Verification items for the finished model (mm, model axes). A direction names the side the tool comes from. Round coordinates to 2 decimals unless told otherwise and drop trailing zeros. Write each loop counter-clockwise with the first axis right and the second up, starting at its lowest first coordinate (ties: lowest second). Pieces come first, ordered by that corner, then holes. Notation, with made-up numbers: (47, 41) - (52, 41) arc R24 ccw to (52, 77) - close; hole circle Ø9 at (20.25, 39.5). An arc over 180 degrees is marked (long way). Write each question's results on one line, items separated by ' | '.
```python
from build123d import *

# Parameters (mm, degrees)
SKETCH1_W               = 25.4
SKETCH1_H               = 10.16
REVOLVE1_ANGLE          = 180
SKETCH4_W               = 6.29000012
SKETCH4_H               = 3.69
SKETCH6_W               = 3.294985449
SKETCH6_H               = 5.974962046
BOSS_EXTRUDE1_DEPTH     = 5.08
SKETCH7_R               = 3.22
BOSS_EXTRUDE7_DEPTH     = 12.7
SKETCH9_W               = 3.294985449
SKETCH9_H               = 5.974962046
BOSS_EXTRUDE8_DEPTH     = 3.302
CUT_EXTRUDE1_DEPTH      = 3.302
CUT_EXTRUDE1_DEPTH_BACK = 3.302
SKETCH11_R              = 2.375
CUT_EXTRUDE2_DEPTH      = 2.54
CUT_EXTRUDE2_DEPTH_BACK = 12.446
BOSS_EXTRUDE14_DEPTH    = 3.81
SKETCH15_R              = 2.375
CUT_EXTRUDE3_DEPTH      = 22.352


with BuildPart() as part:
    # Sketch1 → Revolve1 (revolve)
    with BuildSketch(Plane(origin=(0, 0, 0), x_dir=(1, 0, 0), z_dir=(0, 1, 0))):
        with Locations((12.7, 5.451011236)):
            Rectangle(SKETCH1_W, SKETCH1_H)
    revolve(axis=Axis((0, 0, -0.371011236), (1, 0, 0)), revolution_arc=REVOLVE1_ANGLE)

    # Sweep1: sweep along a path in Sketch5
    with BuildLine(Plane.XY) as sweep1_path:
        ThreePointArc((12.7, 0), (20.315428689, -15.331843414), (12.392600359, -30.5071183))
    # Sketch4 → Sweep1 (sweep)
    with BuildSketch(Plane(origin=(0, 0, 0), x_dir=(1, 0, 0), z_dir=(0, 1, 0))):
        with Locations((12.7, 0.371011236)):
            Rectangle(SKETCH4_W, SKETCH4_H)
    sweep(path=sweep1_path.line)

    # Sketch6 → Boss-Extrude1 (add)
    with BuildSketch(Plane(origin=(20.164340987, -6.538110874, 0), x_dir=(0, 0, 1), z_dir=(-0.95124601, 0.308433183, 0))):
        with Locations((-0.361104817, -25.204906835)):
            Rectangle(SKETCH6_W, SKETCH6_H)
    extrude(amount=BOSS_EXTRUDE1_DEPTH)

    # Sketch7 → Boss-Extrude7 (add)
    with BuildSketch(Plane(origin=(15.332011256, -4.971270302, 0), x_dir=(0, 0, 1), z_dir=(-0.95124601, 0.308433183, 0))):
        with Locations((-0.361104816, -31.160979548)):
            Circle(SKETCH7_R)
    extrude(amount=-BOSS_EXTRUDE7_DEPTH)

    # Sketch9 → Boss-Extrude8 (add)
    with BuildSketch(Plane(origin=(15.332011256, -4.971270302, 0), x_dir=(0, 0, 1), z_dir=(-0.95124601, 0.308433183, 0))):
        with Locations((-0.361104817, -25.204906835)):
            Rectangle(SKETCH9_W, SKETCH9_H)
    extrude(amount=BOSS_EXTRUDE8_DEPTH)

    # Sketch10 → Cut-Extrude1 (cut, two sides)
    with BuildSketch(Plane.XY) as cut_extrude1_sk:
        with BuildLine():
            Line((3.495528998, -30.770720391), (5.338405562, -25.087061585))
            Line((5.338405562, -25.087061585), (13.311749617, -27.672348528))
            add(Edge.make_bspline(
                [(13.311749617, -27.672348528), (8.683653097, -30.129373505), (3.495528998, -30.770720391)],
                knots=[0, 0, 0, 1, 1, 1], degree=2))
        make_face()
    extrude(amount=CUT_EXTRUDE1_DEPTH, mode=Mode.SUBTRACT)
    extrude(cut_extrude1_sk.sketch, amount=-CUT_EXTRUDE1_DEPTH_BACK, mode=Mode.SUBTRACT)

    # Sketch11 → Cut-Extrude2 (cut, two sides)
    with BuildSketch(Plane(origin=(27.412835582, -8.888371731, 0), x_dir=(0, 0, -1), z_dir=(0.95124601, -0.308433183, 0))) as cut_extrude2_sk:
        with Locations((0.39169909, -31.12675273)):
            Circle(SKETCH11_R)
    extrude(amount=CUT_EXTRUDE2_DEPTH, mode=Mode.SUBTRACT)
    extrude(cut_extrude2_sk.sketch, amount=-CUT_EXTRUDE2_DEPTH_BACK, mode=Mode.SUBTRACT)

    # Sketch13 → Boss-Extrude14 (add)
    with BuildSketch(Plane(origin=(27.412835582, -8.888371731, 0), x_dir=(0, 0, -1), z_dir=(0.95124601, -0.308433183, 0))):
        with BuildLine():
            Line((6.519856112, -42.694953789), (3.125271975, -32.910924296))
            Line((3.125271975, -32.910924296), (0.972674671, -34.333593678))
            Line((0.972674671, -34.333593678), (4.157973921, -43.514412461))
            ThreePointArc((4.157973921, -43.514412461), (4.274214649, -43.645179802), (4.448875729, -43.655451668))
            Line((4.448875729, -43.655451668), (6.378816905, -42.985855597))
            ThreePointArc((6.378816905, -42.985855597), (6.509584246, -42.869614869), (6.519856112, -42.694953789))
        make_face()
        with BuildLine():
            Line((4.098849122, -37.242411221), (5.662835166, -41.750205096))
            ThreePointArc((5.662835166, -41.750205096), (5.6525633, -41.924866176), (5.521795959, -42.041106905))
            Line((5.521795959, -42.041106905), (4.53660766, -42.382919506))
            ThreePointArc((4.53660766, -42.382919506), (4.361946579, -42.37264764), (4.245705851, -42.241880299))
            Line((4.245705851, -42.241880299), (2.681719808, -37.734086425))
            Line((2.681719808, -37.734086425), (4.098849122, -37.242411221))
        make_face(mode=Mode.SUBTRACT)
    extrude(amount=-BOSS_EXTRUDE14_DEPTH)

    # Sketch15 → Cut-Extrude3 (cut)
    with BuildSketch(Plane(origin=(27.412835582, -8.888371731, 0), x_dir=(0, 0, -1), z_dir=(0.95124601, -0.308433183, 0))):
        with Locations((0.39169909, -31.12675273)):
            Circle(SKETCH15_R)
    extrude(amount=-CUT_EXTRUDE3_DEPTH, mode=Mode.SUBTRACT)


solid = part.part
```
(1) Set-up check for faces 4 (the flat face through (5.06, -36.65, 1.02)), 5 (the cylindrical face through (12.696, -48.188, -5.654)), 6 (the flat face through (10, -31, -2.009)), 7 (the flat face through (10, -31, 1.286)): record each of +Z, -Z, +X, -X, +Y, -Y from which the full face is reachable in a straight line by a thin tool's end or side.
Answer:
face 4: +Z, -Z, -X | face 5: none | face 6: -Z | face 7: +Z
(2) Section check B-B (x = 8). State how many separate pieces and enclosed holes the cut face has, plus the area to 3 significant figures.
Answer:
separate pieces: 2 | enclosed holes: 1 | area: 185 mm2
(3) Go/stop test with flat-tipped pins: pin 1 Ø1 at (x, z) = (23, 4.5) entering from -Y; pin 2 Ø12 at (x, z) = (3.5, 3.5) entering from -Y; pin 3 Ø1.5 at (x, y) = (21.5, -14.5) entering from -Z. Record where each tip stops, or that it passes through.
Answer:
pin 1: y = 0 | pin 2: y = -38.85 | pin 3: z = -2.22
(4) Thickness scan on L1, parallel to Y at x = 16.75, z = 0.5; L2, parallel to Y at x = 15.25, z = 0.5; L3, parallel to Y at x = 6, z = 0.5. Record the ranges inside material, lowest first.
Answer:
L1: -41.45 to -40.47, -35.84 to -34.93, -29.37 to -22.95, -7.33 to -0.91, 0 to 10.12 | L2: -40.96 to -39.98, -35.35 to -34.44, -30.83 to -25.37, -4.91 to 10.12 | L3: -37.97 to -36.98, -31.58 to -30.35, 0 to 10.12
(5) Section check D-D (y = -23.5). Record the cut outline in (x, z).
Answer:
outline: (16.46, -2.22) - (20.6, -2.22) - (20.6, 1.47) - (16.46, 1.47) - close
(6) Section check C-C (y = -4). Record the cut outline in (x, z).
Answer:
outline: (14.52, -2.22) - (19.12, -2.22) - (19.12, 1.47) - (14.52, 1.47) - close
(7) Mould release check, pull along Z, two halves, no side actions. Record for faces 1 (the flat face through (14.06, -43.97, -3.38)), 2 (the flat face through (16.56, -42.36, -2.16)), 3 (the cylindrical face through (12.878, 10.158, -0.594)): released by +Z, released by -Z, zero draft, split by the parting line, or undercut.
Answer:
face 1: undercut | face 2: zero draft | face 3: split by the parting line
(8) Section check A-A (x = 20.5). Record the cut outline in (y, z), plus the area to 3 significant figures.
Answer:
outline: (-23.72, -2.22) - (-6.56, -2.22) - (-6.56, 1.47) - (-23.72, 1.47) - close; (0, -10.53) arc R10.16 ccw to (0, 9.79) - close | area: 225 mm2
